Design review of the part built by this model. Coordinates are the model's own, in mm. Coordinates: 2 decimals unless noted, no trailing zeros. Write each loop counter-clockwise with the first axis right and the second up, starting at its lowest first coordinate (ties: lowest second). Pieces come first, ordered by that corner, then holes. Notation, with made-up numbers: (29.5, 83.5) - (69.5, 83.5) arc R8 cw to (69.5, 91.5) - close; hole circle Ø1 at (7.5, 5). An arc over 180 degrees is marked (long way). One line per item, written item: value.
Autodesk Inventor part; units mm, degrees
ref_plane "YZ Plane" through (0, 0, 0) normal (1, 0, 0) x (0, 1, 0)
ref_plane "XZ Plane" through (0, 0, 0) normal (0, 1, 0) x (-1, 0, 0)
ref_plane "XY Plane" through (0, 0, 0) normal (0, 0, 1) x (1, 0, 0)
sketch "Sketch1" plane through (0, 0, 0) normal (0, 0, 1) x (1, 0, 0)
  circle A0 centre (0, 0) radius 19.7
  line L0 (-1.435, 20.8507) -> (-1.435, 21.3507)
  line L1 (1.435, 21.3507) -> (1.435, 20.8507)
  arc A1 (1.435, 21.3507) -> (-1.435, 21.3507) centre (0, 12.6834) ccw
  line L2 (-5.669, 0) -> (4.2057, 0)
  line L3 (0, 24.0978) -> (0, 18.8809)
  line L4 (-1.435, -20.8507) -> (-1.435, -21.3507)
  line L5 (1.435, -21.3507) -> (1.435, -20.8507)
  arc A2 (-1.435, -21.3507) -> (1.435, -21.3507) centre (0, -12.6834) ccw
  arc A3 (-1.435, 20.8507) -> (-1.435, -20.8507) centre (0, 0) ccw
  arc A4 (1.435, -20.8507) -> (1.435, 20.8507) centre (0, 0) ccw
  dimension "d2" = 0.5
  dimension "d3" = 0.5
  dimension "d4" = 2.87
extrude "Extrusion1" add sketch "Sketch1" along normal blind 2.03
properties part number "venti-valve-lock-ring"
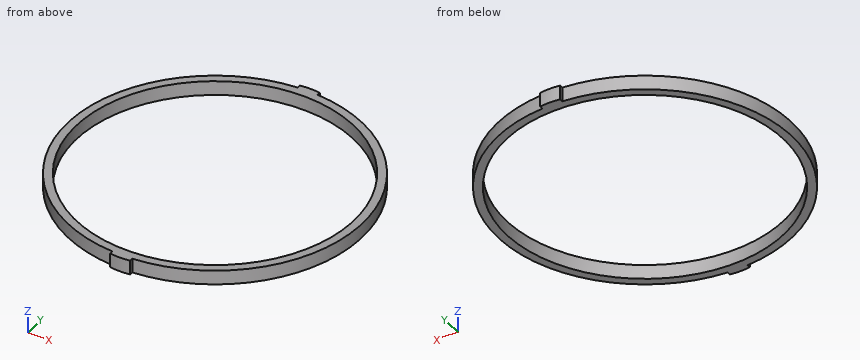
1. Consider section C-C, the plane z = 1.7. Write out the cut boundary in (x, y) (3 decimals).
Answer block:
outline: (-1.435, -21.351) arc R8.785 ccw to (1.435, -21.351) - (1.435, -20.851) arc R20.9 ccw to (1.435, 20.851) - (1.435, 21.351) arc R8.785 ccw to (-1.435, 21.351) - (-1.435, 20.851) arc R20.9 ccw to (-1.435, -20.851) - close; hole circle Ø39.4 at (0, 0)
2. Wall thickness on line 1 along Y through (x, z) = (0, 1.35); line 2 along X through (y, z) = (-0.5, 0.2); line 3 along X through (y, z) = (-9.5, 1.65): over which ranges is each line inside the solid? List them lowest first.
Answer block:
line 1: y = -21.47 to -19.7, 19.7 to 21.47
line 2: x = -20.89 to -19.69, 19.69 to 20.89
line 3: x = -18.62 to -17.26, 17.26 to 18.62
3. Consider section A-A, the plane x = 0. Write out the cut boundary in (y, z), then the cut area to 3 significant figures.
Answer block:
outline: (-21.47, 0) - (-19.7, 0) - (-19.7, 2.03) - (-21.47, 2.03) - close; (19.7, 0) - (21.47, 0) - (21.47, 2.03) - (19.7, 2.03) - close
area: 7.18 mm^2
4. Consider section B-B, the plane y = 8. Write out the cut boundary in (x, z), then the cut area to 3 significant figures.
Answer block:
outline: (-19.31, 0) - (-18, 0) - (-18, 2.03) - (-19.31, 2.03) - close; (18, 0) - (19.31, 0) - (19.31, 2.03) - (18, 2.03) - close
area: 5.30 mm^2
